```python
from build123d import *

# Parameters (mm, degrees)
F0_W     = 50
F0_H     = 50
F1_DEPTH = 25
F2_R     = 10.2048696912
F3_DEPTH = 10
F4_W     = 22.5449811667
F4_H     = 22.3516840488
F5_DEPTH = 25
F6_R     = 5


with BuildPart() as f1:
    # F0 (on Top) → F1 (new body)
    with BuildSketch(Plane.XY):
        with Locations((25, 25)):
            Rectangle(F0_W, F0_H)
    extrude(amount=F1_DEPTH)

    # F2 (on face) → F3 (cut)
    with BuildSketch(Plane.XY.offset(25)):
        with Locations((27.4550188333, 22.3516840488)):
            Circle(F2_R)
    extrude(amount=-F3_DEPTH, mode=Mode.SUBTRACT)

    # F4 (on face) → F5 (cut)
    with BuildSketch(Plane.XY.offset(25)):
        with Locations((38.7275094166, 11.1758420244)):
            Rectangle(F4_W, F4_H)
    extrude(amount=-F5_DEPTH, mode=Mode.SUBTRACT)

    # F6
    f6_edges = [f1.edges().sort_by_distance(p)[0] for p in [
        (0, 25, 25),
        (0, 0, 12.5),
        (13.727509, 0, 0),
        (27.455019, 0, 12.5),
        (13.727509, 0, 25),
        (50, 36.175842, 25),
        (50, 50, 12.5),
        (50, 36.175842, 0),
        (50, 22.351684, 12.5),
    ]]
    fillet(f6_edges, radius=F6_R)


solid = f1.part
```
Here's how the part is built. I have some questions about the finished solid (model axes, mm). A direction names the side the tool comes from. Coordinates: 2 decimals unless noted, no trailing zeros. Loops run counter-clockwise (first coordinate to the right, second up) from the corner with the lowest first, then second, coordinate; pieces in that order, holes last. Notation, with made-up numbers: M 32,82 L 71,82 A27 cw 71,103 Z; hole C 0,47.5 d10. An arc over 180 degrees is marked long. One line per item, written item: value.
1. Imagine slicing it at C-C (x = 37). List the corners of the cut face in (y, z) for me.
Geometry says:
outline: M 22.35,0 L 50,0 L 50,25 L 25.96,25 L 25.96,15 L 22.35,15 Z
2. On a 3-axis mill with a long thin cutter (end or side, diameter ignored), from which of +Z, -Z, +X, -X, +Y, -Y can I reach the whole of each face in a straight line? I mean faces 4 (the flat face through (27.455, 12, 10)), 5 (the flat face through (14, 0, 12)), 6 (the flat face through (27, 22, 15)). Say none if no direction works.
Geometry says:
face 4: +Z, -Z, +X, -Y
face 5: +Z, -Z, +X, -X, -Y
face 6: +Z
3. Please list where these lines run through material, in increasing order: probe 1 along X at (y, z) = (9.5, 4); probe 2 along Y at (x, z) = (44.5, 20.5); probe 3 along Z at (x, y) = (36, 26).
Geometry says:
probe 1: x = 0 to 27.46
probe 2: y = 22.35 to 50
probe 3: z = 0 to 15
4. Will these pins go through, and if not, where does the flat tip stop? pin 1 Ø6 at (y, z) = (23.5, 3.5) entering from +X; pin 2 Ø9 at (x, z) = (40, 18.5) entering from -Y; pin 3 Ø2 at (y, z) = (17, 22) entering from -X.
Geometry says:
pin 1: stops at x = 49.92
pin 2: stops at y = 22.35
pin 3: stops at x = 0.1
5. Thinking about a two-plate mould opening in X: for faces 1 (the cylindrical face through (20.48, 29.8, 20.07)), 2 (the flat face through (0, 27, 10)), 3 (the cylindrical face through (25.951, 1.426, 12.325)), which applies, +X half, -X half, draft (parallel to the pull), parting line (faces both ways), or undercut?
Geometry says:
face 1: undercut
face 2: -X half
face 3: +X half
6. Imagine slicing it at B-B (y = 30). List the corners of the cut face in (x, z) for me.
Geometry says:
outline: M 0,0 L 45,0 A5 ccw 50,5 L 50,20 A5 ccw 45,25 L 34.21,25 L 34.21,15 L 20.7,15 L 20.7,25 L 5,25 A5 ccw 0,20 Z
7. Imagine slicing it at A-A (z = 11). List the corners of the cut face in (x, y) for me, and give its area (3 significant figures).
Geometry says:
outline: M 0,5 A5 ccw 5,0 L 22.46,0 A5 ccw 27.46,5 L 27.46,22.35 L 45,22.35 A5 ccw 50,27.35 L 50,45 A5 ccw 45,50 L 0,50 Z
area: 1,970 mm2
8. Imagine slicing it at D-D (z = 20.75). List the corners of the cut face in (x, y) for me.
Geometry says:
outline: M 0.06,5 A4.94 ccw 5,0.06 L 23.21,0.06 A5 ccw 27.46,5 L 27.46,12.15 A10.2 cw long 37.66,22.35 L 45,22.35 A5 ccw 49.94,26.6 L 49.94,45.75 A5 ccw 45,50 L 0.06,50 Z
